Design review of the part shown in the three views and the two pictorial views. Dimensions are in mm from the part's minimum x, y and z. A direction names the side the tool comes from. Coordinates: 2 decimals unless noted, no trailing zeros. Order: outer loops, then holes, each group sorted by start corner. A loop starts at its lowest first (then second) coordinate and runs counter-clockwise, first axis right, second up. Notation, with made-up numbers: (68.25, -25.75) - (101.25, -25.75) arc R19 ccw to (101.25, 8.25) - close; hole circle Ø8 at (54, 79). An arc over 180 degrees is marked (long way). One line per item, written item: value. Start each with the question number.
(1) Clearance check with a flat-ended pin moving along its axis: pin 1 (7.5 mm diameter, centred on x = 34.5, y = 24, fed in from +Z). State where the tip first meets the part, or that it passes through.
(2) Consider section C-C on z = 17.5. Write out the cut boundary in (x, y), then the cut area to 3 significant figures.
(3) Consider section B-B on x = 31. Write out the cut boundary in (y, z), then the cut area to 3 significant figures.
(4) Mouldability with a two-part tool opening along X and no side actions: class the marked faces 1, 2 and 3 as released by +X, released by -X, zero draft, split by the parting line, or undercut.
(5) For the marked faces 4 and 5, list the 3-axis set-ups (+Z, -Z, +X, -X, +Y, -Y) from which the entire face can be reached by the end or side of a thin tool; tool diameter is ignored.
(6) To check wall thickness, follow line 1 along X through (y, z) = (31.5, 15); line 2 along Y through (x, z) = (47, 16.25); line 3 along Z through (x, y) = (26, 18.5). State the ranges of each line that lie inside material, in increasing order.
(7) Consider section A-A on y = 30. Write out the cut boundary in (x, z).
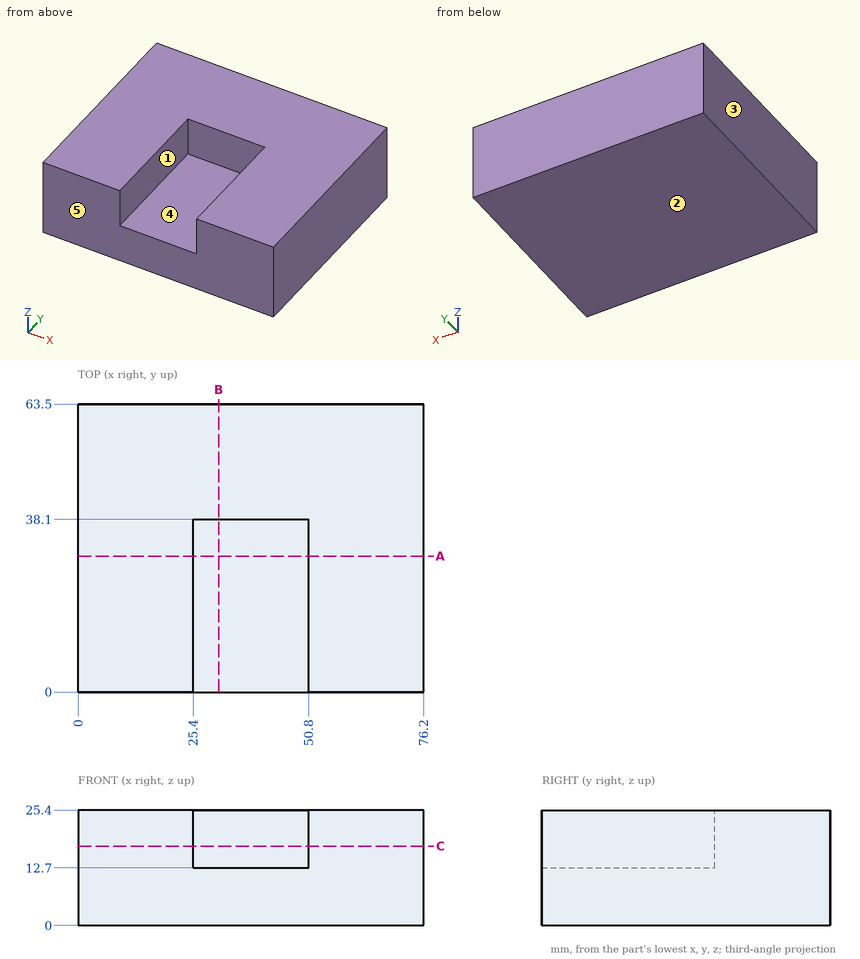
Geometry check:
1. pin 1: stops at z = 12.7
2. outline: (0, 0) - (25.4, 0) - (25.4, 38.1) - (50.8, 38.1) - (50.8, 0) - (76.2, 0) - (76.2, 63.5) - (0, 63.5) - close
2. area: 3,870 mm^2
3. outline: (0, 0) - (63.5, 0) - (63.5, 25.4) - (38.1, 25.4) - (38.1, 12.7) - (0, 12.7) - close
3. area: 1,130 mm^2
4. face 1: undercut
4. face 2: zero draft
4. face 3: released by -X
5. face 4: +Z, -Y
5. face 5: +Z, -Z, +X, -X, -Y
6. line 1: x = 0 to 25.4, 50.8 to 76.2
6. line 2: y = 38.1 to 63.5
6. line 3: z = 0 to 12.7
7. outline: (0, 0) - (76.2, 0) - (76.2, 25.4) - (50.8, 25.4) - (50.8, 12.7) - (25.4, 12.7) - (25.4, 25.4) - (0, 25.4) - close
